For this review, take the finished solid that the model builds, in its own axes (mm). Face numbers are marked on the shaded views. A direction names the side the tool comes from. Give positions to 0.01 mm unless a question says otherwise; leave off trailing zeros. Loops run counter-clockwise (first coordinate to the right, second up) from the corner with the lowest first, then second, coordinate; pieces in that order, holes last. Notation, with made-up numbers: (89, -2) - (103, -2) arc R26 ccw to (103, 30) - close; hole circle Ø2 at (66.25, 50). An arc over 180 degrees is marked (long way). Answer in a Markdown table with one row per item.
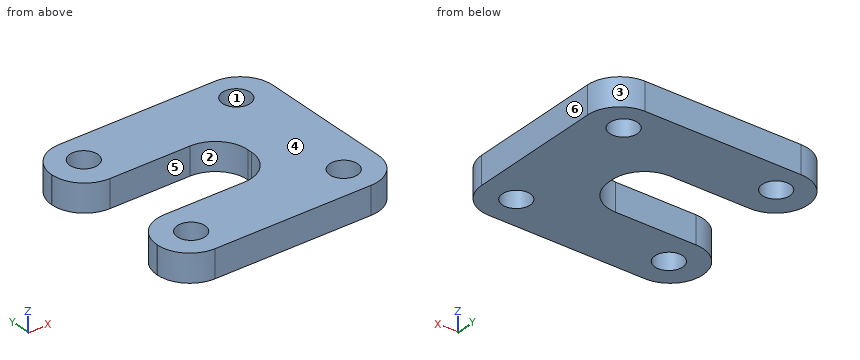
```python
from build123d import *

# Parameters (mm, degrees)
BOSS_EXTRUDE1_DEPTH = 6
SKETCH2_R           = 3
CUT_EXTRUDE1_DEPTH  = 10


with BuildPart() as part:
    # Sketch1 → Boss-Extrude1 (new body)
    with BuildSketch(Plane.XY):
        with BuildLine():
            Line((-96.675181291, 41.529422732), (-96.675181291, 41.429422732))
            ThreePointArc((-96.675181291, 41.429422732), (-94.62492876, 36.479675264), (-89.675181291, 34.429422732))
            Line((-89.675181291, 34.429422732), (-72.346473379, 34.429422732))
            ThreePointArc((-72.346473379, 34.429422732), (-67.396725911, 32.379170201), (-65.346473379, 27.429422732))
            Line((-65.346473379, 27.429422732), (-65.346473379, 26.429422732))
            ThreePointArc((-65.346473379, 26.429422732), (-67.396725911, 21.479675264), (-72.346473379, 19.429422732))
            Line((-72.346473379, 19.429422732), (-89.675181291, 19.429422732))
            ThreePointArc((-89.675181291, 19.429422732), (-94.62492876, 17.379170201), (-96.675181291, 12.429422732))
            Line((-96.675181291, 12.429422732), (-96.675181291, 12.329422732))
            ThreePointArc((-96.675181291, 12.329422732), (-94.62492876, 7.379675264), (-89.675181291, 5.329422732))
            Line((-89.675181291, 5.329422732), (-55.978821898, 5.329422732))
            ThreePointArc((-55.978821898, 5.329422732), (-51.02907443, 7.379675264), (-48.978821898, 12.329422732))
            Line((-48.978821898, 12.329422732), (-48.978821898, 41.529422732))
            ThreePointArc((-48.978821898, 41.529422732), (-51.02907443, 46.479170201), (-55.978821898, 48.529422732))
            Line((-55.978821898, 48.529422732), (-89.675181291, 48.529422732))
            ThreePointArc((-89.675181291, 48.529422732), (-94.62492876, 46.479170201), (-96.675181291, 41.529422732))
        make_face()
    extrude(amount=BOSS_EXTRUDE1_DEPTH)

    # Sketch2 → Cut-Extrude1 (cut)
    with BuildSketch(Plane.XY.offset(6)):
        with Locations((-89.385397691, 41.99084206)):
            Circle(SKETCH2_R)
        with Locations((-56.451908776, 41.99084206)):
            Circle(SKETCH2_R)
        with Locations((-56.451908776, 12.329422732)):
            Circle(SKETCH2_R)
        with Locations((-89.385397691, 12.329422732)):
            Circle(SKETCH2_R)
    extrude(amount=-CUT_EXTRUDE1_DEPTH, mode=Mode.SUBTRACT)


solid = part.part
```
1. For the marked faces 5 and 6, list the 3-axis set-ups (+Z, -Z, +X, -X, +Y, -Y) from which the entire face can be reached by the end or side of a thin tool; tool diameter is ignored.
Values:
| item | result |
|---|---|
| face 5 | +Z, -Z, -X |
| face 6 | +Z, -Z, +X, +Y, -Y |
2. We need section C-C, the plane x = -90.5. Give the boundary of the cut face in (y, z).
Values:
| item | result |
|---|---|
| outline | (5.38, 0) - (9.54, 0) - (9.54, 6) - (5.38, 6) - close; (15.11, 0) - (19.38, 0) - (19.38, 6) - (15.11, 6) - close; (34.48, 0) - (39.21, 0) - (39.21, 6) - (34.48, 6) - close; (44.78, 0) - (48.48, 0) - (48.48, 6) - (44.78, 6) - close |
3. Wall thickness on line 1 (X direction, y = 12.5, z = 4.9); line 2 (Y direction, x = -55.5, z = 1.35); line 3 (X direction, y = 42.5, z = 4.4): over which ranges is each line inside the solid? List them lowest first. Write a range as [from, to].
Values:
| item | result |
|---|---|
| line 1 | x = [-96.67, -92.38], [-86.39, -59.45], [-53.46, -48.98] |
| line 2 | y = [5.35, 9.48], [15.17, 39.15], [44.84, 48.51] |
| line 3 | x = [-96.61, -92.34], [-86.43, -59.41], [-53.5, -49.05] |
4. Clearance check with a flat-ended pin moving along its axis: pin 1 (0.5 mm diameter, centred on y = 27, z = 2.5, fed in from -X). State where the tip first meets the part, or that it passes through.
Values:
| item | result |
|---|---|
| pin 1 | stops at x = -65.35 |
5. Mouldability with a two-part tool opening along X and no side actions: class the marked faces 1, 2, 3 and 4 as released by +X, released by -X, zero draft, split by the parting line, or undercut.
Values:
| item | result |
|---|---|
| face 1 | undercut |
| face 2 | released by -X |
| face 3 | released by +X |
| face 4 | zero draft |
6. We need section A-A, the plane x = -75. Give the boundary of the cut face in (y, z).
Values:
| item | result |
|---|---|
| outline | (5.33, 0) - (19.43, 0) - (19.43, 6) - (5.33, 6) - close; (34.43, 0) - (48.53, 0) - (48.53, 6) - (34.43, 6) - close |
7. We need section D-D, the plane x = -57.5. Give the boundary of the cut face in (y, z).
Values:
| item | result |
|---|---|
| outline | (5.33, 0) - (9.52, 0) - (9.52, 6) - (5.33, 6) - close; (15.14, 0) - (39.18, 0) - (39.18, 6) - (15.14, 6) - close; (44.8, 0) - (48.53, 0) - (48.53, 6) - (44.8, 6) - close |
8. We need section B-B, the plane y = 10. Give the boundary of the cut face in (x, z).
Values:
| item | result |
|---|---|
| outline | (-96.28, 0) - (-91.28, 0) - (-91.28, 6) - (-96.28, 6) - close; (-87.49, 0) - (-58.34, 0) - (-58.34, 6) - (-87.49, 6) - close; (-54.56, 0) - (-49.38, 0) - (-49.38, 6) - (-54.56, 6) - close |
